```python
from build123d import *

# Parameters (mm, degrees)
SKETCH9_W           = 35
SKETCH9_H           = 30.5
SKETCH9_W_2         = 9
SKETCH9_H_2         = 9
BOSS_EXTRUDE5_DEPTH = 2
BOSS_EXTRUDE6_DEPTH = 1
CUT_EXTRUDE4_REACH  = 44.474
SKETCH12_R          = 1.25
SKETCH16_W          = 35
SKETCH16_H          = 22
SKETCH16_R          = 2
SKETCH16_W_2        = 28
SKETCH16_H_2        = 10
BOSS_EXTRUDE9_DEPTH = 3
SKETCH17_W          = 31
SKETCH17_H          = 1
CUT_EXTRUDE8_DEPTH  = 47.864165415
FILLET3_R           = 3


with BuildPart() as part:
    # Sketch9 → Boss-Extrude5 (new body)
    with BuildSketch(Plane(origin=(0, 0, 0), x_dir=(1, 0, 0), z_dir=(0, 1, 0))):
        with Locations((12.5, 14.75)):
            Rectangle(SKETCH9_W, SKETCH9_H)
        with Locations((12.5, 9.5)):
            Rectangle(SKETCH9_W_2, SKETCH9_H_2, mode=Mode.SUBTRACT)
    extrude(amount=BOSS_EXTRUDE5_DEPTH)

    # Sketch10 → Boss-Extrude6 (add)
    with BuildSketch(Plane(origin=(0, 2, 0), x_dir=(1, 0, 0), z_dir=(0, 1, 0))):
        Polygon((28, -0.5), (28, 28), (-3, 28), (-3, -0.5), (-5, -0.5), (-5, 30), (30, 30), (30, -0.5), align=None)
    extrude(amount=BOSS_EXTRUDE6_DEPTH)

    # Sketch12 → Cut-Extrude4 (cut, up to next)
    with BuildSketch(Plane(origin=(0, 2, 0), x_dir=(1, 0, 0), z_dir=(0, 1, 0)), mode=Mode.PRIVATE) as cut_extrude4_sk1:
        with Locations(Location((2, 22, 0), (0, 0, 270))):
            Circle(SKETCH12_R)
    cut_extrude4_tool1 = extrude(cut_extrude4_sk1.sketch, amount=-CUT_EXTRUDE4_REACH, mode=Mode.PRIVATE) & part.part
    # Sketch12 → Cut-Extrude4 (cut, up to next)
    with BuildSketch(Plane(origin=(0, 2, 0), x_dir=(1, 0, 0), z_dir=(0, 1, 0)), mode=Mode.PRIVATE) as cut_extrude4_sk2:
        with Locations(Location((2, 9.5, 0), (0, 0, 270))):
            Circle(SKETCH12_R)
    cut_extrude4_tool2 = extrude(cut_extrude4_sk2.sketch, amount=-CUT_EXTRUDE4_REACH, mode=Mode.PRIVATE) & part.part
    # Sketch12 → Cut-Extrude4 (cut, up to next)
    with BuildSketch(Plane(origin=(0, 2, 0), x_dir=(1, 0, 0), z_dir=(0, 1, 0)), mode=Mode.PRIVATE) as cut_extrude4_sk3:
        with Locations(Location((23, 9.5, 0), (0, 0, 270))):
            Circle(SKETCH12_R)
    cut_extrude4_tool3 = extrude(cut_extrude4_sk3.sketch, amount=-CUT_EXTRUDE4_REACH, mode=Mode.PRIVATE) & part.part
    # Sketch12 → Cut-Extrude4 (cut, up to next)
    with BuildSketch(Plane(origin=(0, 2, 0), x_dir=(1, 0, 0), z_dir=(0, 1, 0)), mode=Mode.PRIVATE) as cut_extrude4_sk4:
        with Locations(Location((23, 22, 0), (0, 0, 270))):
            Circle(SKETCH12_R)
    cut_extrude4_tool4 = extrude(cut_extrude4_sk4.sketch, amount=-CUT_EXTRUDE4_REACH, mode=Mode.PRIVATE) & part.part
    add(cut_extrude4_tool1.solids().sort_by_distance((2, 2, -22))[0], mode=Mode.SUBTRACT)
    add(cut_extrude4_tool2.solids().sort_by_distance((2, 2, -9.5))[0], mode=Mode.SUBTRACT)
    add(cut_extrude4_tool3.solids().sort_by_distance((23, 2, -9.5))[0], mode=Mode.SUBTRACT)
    add(cut_extrude4_tool4.solids().sort_by_distance((23, 2, -22))[0], mode=Mode.SUBTRACT)

    # Sketch16 → Boss-Extrude9 (add)
    with BuildSketch(Plane.XY.offset(-17.5)):
        with Locations((12.5, 11)):
            Rectangle(SKETCH16_W, SKETCH16_H)
        with Locations((0.5, 18)):
            Circle(SKETCH16_R, mode=Mode.SUBTRACT)
        with Locations(Location((24.5, 18, 0), (0, 0, 180))):
            Circle(SKETCH16_R, mode=Mode.SUBTRACT)
        with Locations((12.5, 7)):
            Rectangle(SKETCH16_W_2, SKETCH16_H_2, mode=Mode.SUBTRACT)
    extrude(amount=BOSS_EXTRUDE9_DEPTH)

    # Sketch17 → Cut-Extrude8 (cut, through all)
    with BuildSketch(Plane.XY.offset(-28)):
        with Locations((12.5, 2.5)):
            Rectangle(SKETCH17_W, SKETCH17_H)
    extrude(amount=-CUT_EXTRUDE8_DEPTH, mode=Mode.SUBTRACT)

    # Fillet3
    fillet3_edges = [part.edges().sort_by_distance(p)[0] for p in [
        (-4, 3, -17.5),
        (29, 3, -17.5),
        (-4, 3, -14.5),
        (29, 3, -14.5),
        (-5, 22, -16),
        (30, 22, -16),
    ]]
    fillet(fillet3_edges, radius=FILLET3_R)


solid = part.part
```
Source: CAD feature listing. Evaluate the final solid. Frame: model axes, mm. A direction names the side the tool comes from. Round coordinates to 2 decimals unless told otherwise and drop trailing zeros. Loops run counter-clockwise (first coordinate to the right, second up) from the corner with the lowest first, then second, coordinate; pieces in that order, holes last.
(1) Section query D-D (y = 3.75). Output: boundary loops of the cut face in (x, z), and give its area (3 significant figures).
From the geometry:
outline: (-5, -18.52) - (-3, -18.52) - (-3, -17.5) - (-1.5, -17.5) - (-1.5, -14.5) - (-3, -14.5) - (-3, -13.48) - (-5, -13.48) - close; (26.5, -17.5) - (28, -17.5) - (28, -18.52) - (30, -18.52) - (30, -13.48) - (28, -13.48) - (28, -14.5) - (26.5, -14.5) - close
area: 29.1 mm2
(2) Contact query for flat-ended pins moving along their axis: pin 1 Ø1.6 at (x, z) = (29, -5.5) entering from +Y; pin 2 Ø6 at (x, y) = (15.5, 8.5) entering from -Z; pin 3 Ø1.5 at (x, y) = (23.5, 19.5) entering from -Z; pin 4 Ø6 at (x, y) = (10.5, 15.5) entering from +Z. Output: stop coordinate, or through.
From the geometry:
pin 1: stops at y = 3
pin 2: passes through
pin 3: stops at z = -17.5
pin 4: stops at z = -14.5
(3) Material intervals for probe 1 along X at (y, z) = (0.7, -9.5); probe 2 along Y at (x, z) = (24.5, -15.4); probe 3 along Z at (x, y) = (-2, 3.25), sorted ascending.
From the geometry:
probe 1: x = -5 to 0.75, 3.25 to 8, 17 to 21.75, 24.25 to 30
probe 2: y = 0 to 2, 12 to 16, 20 to 22
probe 3: z = -17.5 to -14.5
(4) Section query C-C (y = 18.5). Output: boundary loops of the cut face in (x, z), and give its area (3 significant figures).
From the geometry:
outline: (-5, -17.5) - (-1.44, -17.5) - (-1.44, -14.5) - (-5, -14.5) - close; (2.44, -17.5) - (22.56, -17.5) - (22.56, -14.5) - (2.44, -14.5) - close; (26.44, -17.5) - (30, -17.5) - (30, -14.5) - (26.44, -14.5) - close
area: 81.8 mm2
(5) Pull-direction query (X, two-part tool) for faces 6 (the flat face through (12, 0, -15)), 7 (the cylindrical face through (0.24, 19.983, -16.021)); classes: +X half, -X half, draft (parallel to the pull), parting line (faces both ways), or undercut.
From the geometry:
face 6: draft
face 7: undercut
(6) Section query A-A (z = -9.5). Output: boundary loops of the cut face in (x, y).
From the geometry:
outline: (-5, 0) - (0.75, 0) - (0.75, 2) - (-3, 2) - (-3, 3) - (-5, 3) - close; (3.25, 0) - (8, 0) - (8, 2) - (3.25, 2) - close; (17, 0) - (21.75, 0) - (21.75, 2) - (17, 2) - close; (24.25, 0) - (30, 0) - (30, 3) - (28, 3) - (28, 2) - (24.25, 2) - close
(7) Section query B-B (x = 12). Output: boundary loops of the cut face in (y, z), and give its area (3 significant figures).
From the geometry:
outline: (0, -30) - (2, -30) - (2, -14) - (0, -14) - close; (0, -5) - (2, -5) - (2, 0.5) - (0, 0.5) - close; (12, -17.5) - (22, -17.5) - (22, -14.5) - (12, -14.5) - close
area: 73.0 mm2
(8) Access query for faces 1 (the flat face through (26.5, 7, -16)), 2 (the flat face through (28, 2.7, -22.8)), 3 (the flat face through (12, 1, -5)), 4 (the flat face through (-3, 2.7, -7.6)), 5 (the flat face through (-4, 3, -6)). Directions: +Z, -Z, +X, -X, +Y, -Y. A direction counts if a zero-diameter tool reaches every point of the face in a straight line with its end or side. Return the directions, or none.
From the geometry:
face 1: +Z, -Z
face 2: -Z, +Y
face 3: +Y, -Y
face 4: +Z, +Y
face 5: +Z, +X, -X, +Y
